Geometry check sheet. Reference: drawing and pictorial views, mm from the part's lowest x, y, z. Give positions to 0.01 mm unless a question says otherwise; leave off trailing zeros. Order: outer loops, then holes, each group sorted by start corner. A loop starts at its lowest first (then second) coordinate and runs counter-clockwise, first axis right, second up.
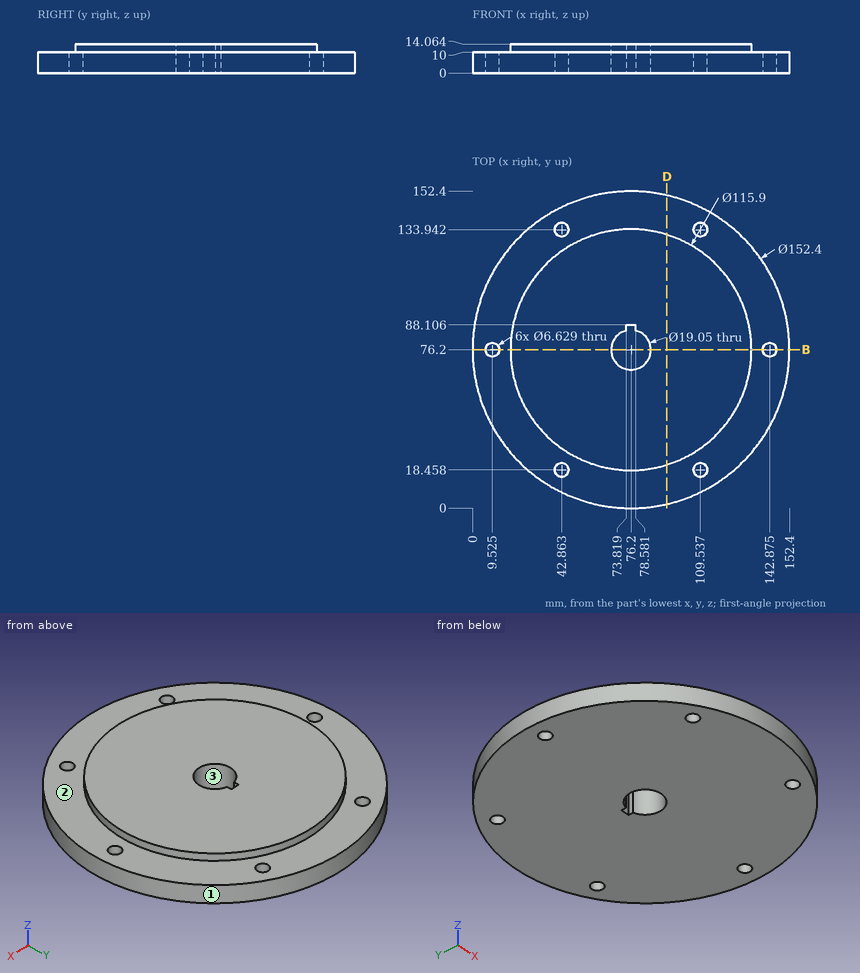
1) Depth check by flat-ended pin: pin 1 Ø3 at (x, z) = (32.5, 4.5) entering from +Y; pin 2 Ø10.5 at (x, y) = (109.54, 18.46) entering from +Z; pin 3 Ø2 at (y, z) = (86.5, 7) entering from +X. Enter the tip coordinate at first touch or a pass-through.
Recorded:
pin 1: stops at y = 139.65
pin 2: stops at z = 10
pin 3: stops at x = 151.83
2) Section check D-D, the plane x = 93.5. Record the cut outline in (y, z) (1 decimal), then the cut area to 3 significant figures.
Recorded:
outline: (2, 0) - (150.4, 0) - (150.4, 10) - (131.5, 10) - (131.5, 14.1) - (20.9, 14.1) - (20.9, 10) - (2, 10) - close
area: 1,930 mm2
3) Section check B-B, the plane y = 76.2. State how many separate pieces and enclosed holes the cut face has, then the cut area to 3 significant figures.
Recorded:
separate pieces: 4
enclosed holes: 0
area: 1,590 mm2
4) Material ranges on L1, parallel to Y at x = 45, z = 1.75 (1 decimal); L2, parallel to Z at x = 136.5, y = 44.5; L3, parallel to Y at x = 111.5, z = 7.5 (1 decimal), recorded low to high.
Recorded:
L1: y = 6.7 to 15.9, 21 to 131.4, 136.5 to 145.7
L2: z = 0 to 10
L3: y = 8.7 to 15.8, 21.1 to 131.3, 136.6 to 143.7
5) Draft check along X on the marked faces 1, 2 and 3. Enter one of: +X half, -X half, draft (parallel to the pull), parting line (faces both ways), or undercut.
Recorded:
face 1: parting line
face 2: draft
face 3: undercut
